Can you work these out from the model? Positions are in its coordinate system, mm. Face numbers are marked on the shaded views. A direction names the side the tool comes from. Give positions to 0.01 mm unless a question says otherwise; leave off trailing zeros. Loops run counter-clockwise (first coordinate to the right, second up) from the corner with the lowest first, then second, coordinate; pieces in that order, holes last. Notation, with made-up numbers: M 67,-19.5 L 122,-19.5 A14 ccw 122,-7.5 Z; hole C 69,51.5 d6. An arc over 180 degrees is marked long. Answer as a JSON object with one key per item and string values.
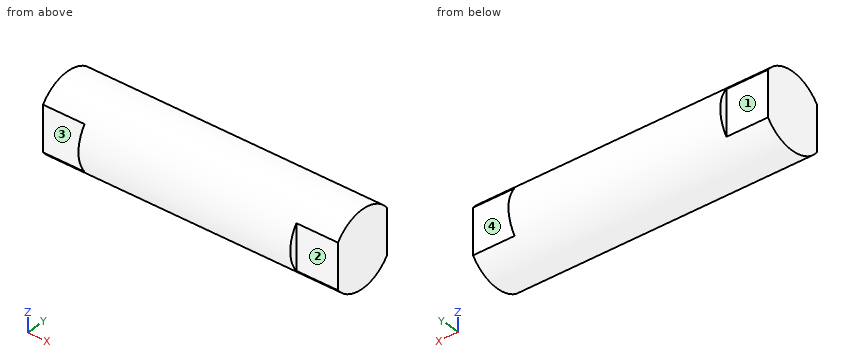
```python
from build123d import *

# Parameters (mm, degrees)
SKETCH1_R           = 2.5
BOSS_EXTRUDE1_DEPTH = 9.75
CUT_EXTRUDE1_START  = -2.749999999
CUT_EXTRUDE1_DEPTH  = 2.749999999


with BuildPart() as part:
    # Sketch1 → Boss-Extrude1 (new, symmetric)
    with BuildSketch(Plane(origin=(0, 0, 0), x_dir=(0, 0, -1), z_dir=(1, 0, 0))):
        with Locations(Location((0, 0, 0), (0, 0, 180))):
            Circle(SKETCH1_R)
    extrude(amount=BOSS_EXTRUDE1_DEPTH, both=True)

    # Sketch2 → Cut-Extrude1 (cut)
    with BuildSketch(Plane.ZY.offset(9.75).offset(CUT_EXTRUDE1_START)):
        with BuildLine():
            Line((-1.5, 2), (1.5, 2))
            ThreePointArc((1.5, 2), (0, 2.5), (-1.5, 2))
        make_face()
        with BuildLine():
            Line((1.5, -2), (-1.5, -2))
            ThreePointArc((-1.5, -2), (0, -2.5), (1.5, -2))
        make_face()
    cut_extrude1 = extrude(amount=CUT_EXTRUDE1_DEPTH, mode=Mode.SUBTRACT)

    # Mirror1: Cut-Extrude1 across plane
    add(cut_extrude1.mirror(Plane(origin=(0, 0, 0), x_dir=(0, 0, 1), z_dir=(1, 0, 0))), mode=Mode.SUBTRACT)


solid = part.part
```
1) Suppose I cut it at C-C, the plane y = 1.7. Write out the boundary of the cut face in (x, z), and give its area (3 significant figures).
Answer list:
{"outline": "M -9.75,-1.83 L 9.75,-1.83 L 9.75,1.83 L -9.75,1.83 Z", "area": "71.5 mm^2"}
2) For the marked faces 1, 2, 3 and 4, which set-ups out of +Z, -Z, +X, -X, +Y, -Y let a thin tool reach every point of the face, with its end or its side?
Answer list:
{"face 1": "+Z, -Z, -X, +Y", "face 2": "+Z, -Z, +X, -Y", "face 3": "+Z, -Z, -X, -Y", "face 4": "+Z, -Z, +X, +Y"}
3) Suppose I cut it at B-B, the plane x = -4.5. Write out the boundary of the cut face in (y, z), and give its area (3 significant figures).
Answer list:
{"outline": "C 0,0 d5", "area": "19.6 mm^2"}
4) Will these pins go through, and if not, where does the flat tip stop? pin 1 Ø3 at (x, z) = (-7.5, -1.5) entering from +Y; pin 2 Ø0.8 at (x, z) = (8, 0.5) entering from -Y; pin 3 Ø2 at (x, z) = (-9, -0.5) entering from +Y.
Answer list:
{"pin 1": "y = 2.5", "pin 2": "y = -2", "pin 3": "y = 2"}
5) Suppose I cut it at A-A, the plane z = 0. Write out the boundary of the cut face in (x, y), and give its area (3 significant figures).
Answer list:
{"outline": "M -9.75,-2 L -7,-2 L -7,-2.5 L 7,-2.5 L 7,-2 L 9.75,-2 L 9.75,2 L 7,2 L 7,2.5 L -7,2.5 L -7,2 L -9.75,2 Z", "area": "92.0 mm^2"}
6) Suppose I cut it at D-D, the plane z = 0.9. Write out the boundary of the cut face in (x, y).
Answer list:
{"outline": "M -9.75,-2 L -7,-2 L -7,-2.33 L 7,-2.33 L 7,-2 L 9.75,-2 L 9.75,2 L 7,2 L 7,2.33 L -7,2.33 L -7,2 L -9.75,2 Z"}
7) Please list where these lines run through material, in increasing order: line 1 along Z through (x, y) = (6.5, 2); line 2 along Y through (x, z) = (8, -0.2). Write a range as from..to.
Answer list:
{"line 1": "-1.5..1.5", "line 2": "-2..2"}
